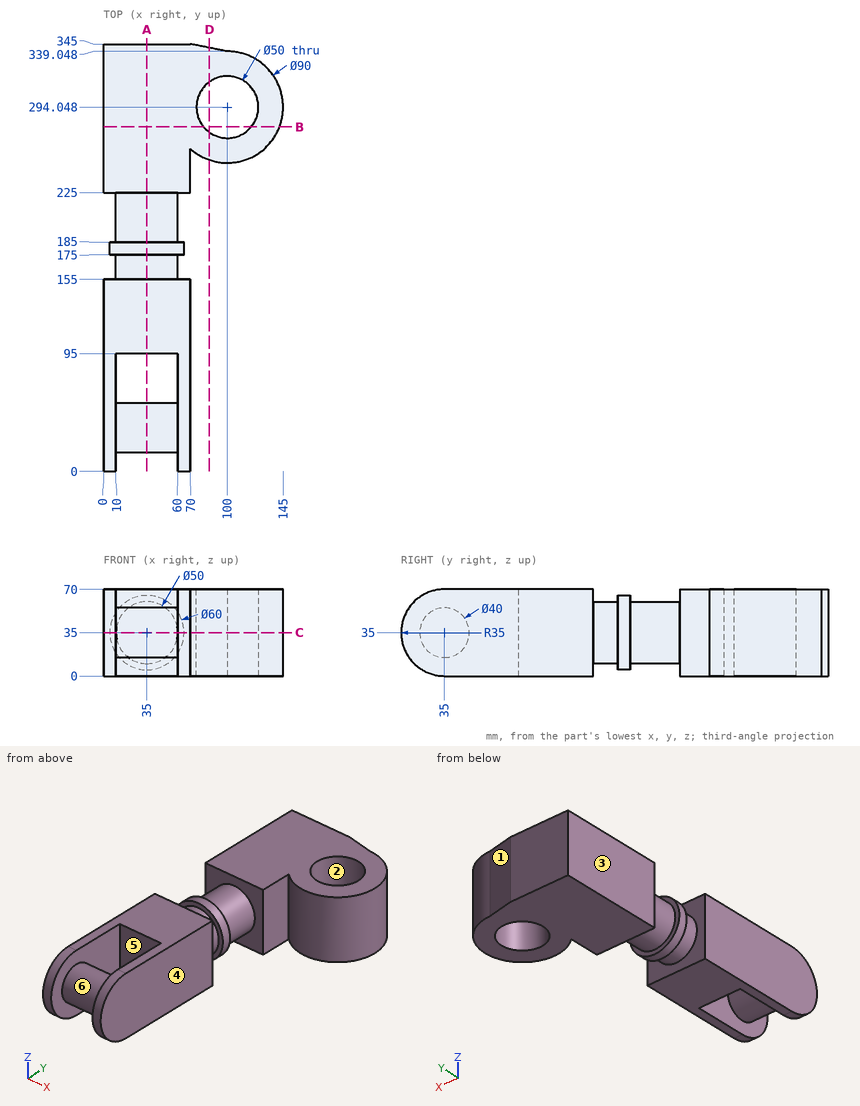
Print and shaded views of the part. All mm, measured from the part's lowest x, y and z. A direction names the side the tool comes from. Coordinates: 2 decimals unless noted, no trailing zeros. Write each loop counter-clockwise with the first axis right and the second up, starting at its lowest first coordinate (ties: lowest second). Pieces come first, ordered by that corner, then holes. Notation, with made-up numbers: (62, 15.5) -> (73, 15.5) arc R6 cw to (73, 22.5) -> close; hole circle Ø9 at (-36.75, -21). An arc over 180 degrees is marked (long way). Use CSV: the item, a comma, the result in double quotes. Start each with the question number.
Q1. 3-axis set-ups, long thin cutter, end or side, ignore diameter. For the marked faces 4, 5 and 6: which of +Z, -Z, +X, -X, +Y, -Y reach the whole face in a straight line?
Q2. Cut at C-C, the plane z = 35. State how many separate pieces and enclosed holes the cut face has, then the cut area to 3 significant figures.
Q3. Drill centre lines: probe 1 along X at (y, z) = (86.5, 9); probe 2 along Y at (x, z) = (22, 63); probe 3 along Y at (x, z) = (100, 50). Where is each one in solid material? Low to high.
Q4. Pull direction X, two halves, no side cores. Call the marked faces 1, 2 and 3: released by +X, released by -X, zero draft, split by the parting line, or undercut.
Q5. Cut at A-A, the plane x = 35. List the corners of the cut face in (y, z).
Q6. Cut at B-B, the plane y = 278. List the corners of the cut face in (x, z), then the cut area to 3 significant figures.
Q7. Cut at D-D, the plane x = 85.5. List the corners of the cut face in (y, z) (1 decimal).
Q8. Flat gauge pins, fed straight in: pin 1 Ø21 at (y, z) = (34.5, 38) entering from +X; pin 2 Ø8 at (y, z) = (173, 13.5) entering from +X; pin 3 Ø3 at (y, z) = (268, 44.5) entering from +X (1 decimal). Where does each tip first touch, or does it go through?
Checked values:
1,face 4,"+Z, -Z, +X, -Y"
1,face 5,"+Z, -Z"
1,face 6,"none"
2,separate pieces,"1"
2,enclosed holes,"2"
2,area,"24,000 mm²"
3,probe 1,"x = 0 to 10, 60 to 70"
3,probe 2,"y = 95 to 155, 225 to 345"
3,probe 3,"y = 249.05 to 269.05, 319.05 to 339.05"
4,face 1,"released by +X"
4,face 2,"undercut"
4,face 3,"released by -X"
5,outline,"circle Ø40 at (35, 35); (95, 0) -> (155, 0) -> (155, 10) -> (175, 10) -> (175, 5) -> (185, 5) -> (185, 10) -> (225, 10) -> (225, 0) -> (345, 0) -> (345, 70) -> (225, 70) -> (225, 60) -> (185, 60) -> (185, 65) -> (175, 65) -> (175, 60) -> (155, 60) -> (155, 70) -> (95, 70) -> close"
6,outline,"(0, 0) -> (80.83, 0) -> (80.83, 70) -> (0, 70) -> close; (119.17, 0) -> (142.04, 0) -> (142.04, 70) -> (119.17, 70) -> close"
6,area,"7,260 mm²"
7,outline,"(251.4, 0) -> (273.7, 0) -> (273.7, 70) -> (251.4, 70) -> close; (314.4, 0) -> (341.9, 0) -> (341.9, 70) -> (314.4, 70) -> close"
8,pin 1,"stops at x = 70"
8,pin 2,"stops at x = 58.97"
8,pin 3,"stops at x = 137.7"
